Could you check a few things on this model? Use its own coordinates, in mm. Give positions to 0.01 mm unless a question says otherwise; leave off trailing zeros. Write each loop counter-clockwise with the first axis right and the second up, starting at its lowest first coordinate (ties: lowest second). Pieces come first, ordered by that corner, then holes. Notation, with made-up numbers: (-2.75, -12.5) - (28.25, -12.5) arc R24 ccw to (28.25, 13.5) - close; hole circle Ø8 at (11, 74.5). An arc over 180 degrees is marked (long way). Answer as CSV lines item,"result". Start each with the question number.
Q1. Imagine slicing it at B-B on x = 22.5. List the corners of the cut face in (y, z) for me.
Q2. We'd pull the mould along X, two halves only. Please class faces 1 (the face through (30, 5, 0)), 2 (the face through (0, 5, -21.5)), 3 (the face through (-23.79, 5.07, -16.18)): pulls with the +X half, pulls with the -X half, needs draft (parallel to the pull), parting line crosses it, or undercut.
Q3. If I drill on line 1 along X through (y, z) = (2.25, 0); line 2 along X through (y, z) = (2.75, 15); line 3 along Z through (x, y) = (22.5, 4), over which ranges is the centre line in solid material (lowest first)?
Q4. Imagine slicing it at C-C on y = 3. List the corners of the cut face in (x, z) for me, and give its area (3 significant figures).
Q5. Imagine slicing it at A-A on z = -15. List the corners of the cut face in (x, y) for me, and give its area (3 significant figures).
Q6. Will this pin go through, and if not, where does the flat tip stop? pin 1 Ø3 at (x, z) = (-22.5, -15) entering from +Y.
```python
from build123d import *

# Parameters (mm, degrees)
SKETCH_2_W          = 60
SKETCH_2_H          = 43
EXTRUDE_1_DEPTH     = 10
SKETCH_3_R          = 1.75
CUT_EXTRUDE_1_DEPTH = 11
SKETCH_4_R          = 1.75
CUT_EXTRUDE_2_DEPTH = 11


with BuildPart() as part:
    # 草图2 → 凸台-拉伸1 (new body)
    with BuildSketch(Plane(origin=(0, 0, 0), x_dir=(1, 0, 0), z_dir=(0, 1, 0))):
        Rectangle(SKETCH_2_W, SKETCH_2_H)
    extrude(amount=EXTRUDE_1_DEPTH)

    # 草图3 → 切除-拉伸1 (cut, through all)
    with BuildSketch(Plane(origin=(0, 10, 0), x_dir=(1, 0, 0), z_dir=(0, 1, 0))):
        with Locations((-22.5, 15)):
            Circle(SKETCH_3_R)
        with Locations((22.5, 15)):
            Circle(SKETCH_3_R)
        with Locations((22.5, -15)):
            Circle(SKETCH_3_R)
        with Locations((-22.5, -15)):
            Circle(SKETCH_3_R)
    extrude(amount=-CUT_EXTRUDE_1_DEPTH, mode=Mode.SUBTRACT)

    # 草图4 → 切除-拉伸2 (cut, through all)
    with BuildSketch(Plane(origin=(0, 10, 0), x_dir=(1, 0, 0), z_dir=(0, 1, 0))):
        with Locations((-20, 0)):
            Circle(SKETCH_4_R)
        with Locations((20, 0)):
            Circle(SKETCH_4_R)
    extrude(amount=-CUT_EXTRUDE_2_DEPTH, mode=Mode.SUBTRACT)


solid = part.part
```
Conclusion:
1,outline,"(0, -21.5) - (10, -21.5) - (10, -16.75) - (0, -16.75) - close; (0, -13.25) - (10, -13.25) - (10, 13.25) - (0, 13.25) - close; (0, 16.75) - (10, 16.75) - (10, 21.5) - (0, 21.5) - close"
2,face 1,"pulls with the +X half"
2,face 2,"needs draft"
2,face 3,"undercut"
3,line 1,"-30 to -21.75, -18.25 to 18.25, 21.75 to 30"
3,line 2,"-30 to -24.25, -20.75 to 20.75, 24.25 to 30"
3,line 3,"-21.5 to -16.75, -13.25 to 13.25, 16.75 to 21.5"
4,outline,"(-30, -21.5) - (30, -21.5) - (30, 21.5) - (-30, 21.5) - close; hole circle Ø3.5 at (-22.5, -15); hole circle Ø3.5 at (-22.5, 15); hole circle Ø3.5 at (-20, 0); hole circle Ø3.5 at (20, 0); hole circle Ø3.5 at (22.5, -15); hole circle Ø3.5 at (22.5, 15)"
4,area,"2,520 mm^2"
5,outline,"(-30, 0) - (-24.25, 0) - (-24.25, 10) - (-30, 10) - close; (-20.75, 0) - (20.75, 0) - (20.75, 10) - (-20.75, 10) - close; (24.25, 0) - (30, 0) - (30, 10) - (24.25, 10) - close"
5,area,"530 mm^2"
6,pin 1,"through"
